Part model, mm, in its own coordinate system. Coordinates: 2 decimals unless noted, no trailing zeros. Order: outer loops, then holes, each group sorted by start corner. A loop starts at its lowest first (then second) coordinate and runs counter-clockwise, first axis right, second up.
1) Cut at A-A (y = 24). List the corners of the cut face in (x, z), and give its area (3 significant figures).
2) Wall check: L1, parallel to X at y = 41, z = -0.75; L2, parallel to Z at x = -0.25, y = 19; L3, parallel to Y at x = -3.25, z = -2.75. Give the ranges that are in metal, low to high.
3) Pin check, flat tips, straight feed: pin 1 Ø3 at (y, z) = (64.5, 1) entering from -X; pin 2 Ø4 at (y, z) = (19.5, -2.5) entering from +X; pin 3 Ø4 at (y, z) = (24.5, 3.5) entering from -X. Stop position of each tip, or through.
```python
from build123d import *

# Parameters (mm, degrees)
FILLET1_R = 2.54
FILLET2_R = 2.54
FILLET3_R = 7.62


with BuildPart() as part:
    # Sketch1 → Revolve1 (revolve)
    with BuildSketch(Plane.XY, mode=Mode.PRIVATE) as revolve1_sk:
        Polygon((0, 0), (1.154700538, 2), (2.660575, 7.62), (3.81, 10.16), (5.08, 10.16), (5.08, 101.6), (0, 101.6), align=None)
    revolve(revolve1_sk.sketch.rotate(Axis((0, 0, 0), (0, 1, 0)), 90), axis=Axis((0, 0, 0), (0, 1, 0)))

    # Fillet1
    # the kernel refuses this fillet: 2.54 mm, written as the material it takes off along each edge
    with BuildSketch(Plane(origin=(0, 10.16, 0), x_dir=(0, 0, -1), z_dir=(1, 0, 0))) as fillet1_piece_1:
        with BuildLine():
            CenterArc((2.54, 2.199704526), FILLET1_R, 300, 60)
            Line((5.08, 2.199704526), (5.1308, 2.199704526))
            Line((5.1308, 2.199704526), (5.1308, 0))
            Line((5.1308, 0), (5.08, -0.0508))
            ThreePointArc((5.08, -0.0508), (4.445, -0.0508), (3.8354, -0.043994091))
            Line((3.8354, -0.043994091), (3.81, 0))
        make_face()
    revolve(axis=Axis((0, 10.16, 0), (0, 1, 0)), mode=Mode.SUBTRACT)

    # Fillet2
    fillet2_edges = [part.edges().sort_by_distance(p)[0] for p in [
        (0, 10.16, 3.81),
    ]]
    fillet(fillet2_edges, radius=FILLET2_R)

    # Fillet3
    fillet3_edges = [part.edges().sort_by_distance(p)[0] for p in [
        (0, 7.62, 2.660575),
        (0, 2, 1.154700538),
    ]]
    fillet(fillet3_edges, radius=FILLET3_R)


solid = part.part
```
Geometry check:
1. outline: circle Ø10.16 at (0, 0)
1. area: 81.1 mm2
2. L1: x = -5.02 to 5.02
2. L2: z = -5.07 to 5.07
2. L3: y = 10.49 to 101.6
3. pin 1: stops at x = -5.08
3. pin 2: stops at x = 5.06
3. pin 3: stops at x = -4.85
